```python
from build123d import *

# Parameters (mm, degrees)
F0_W     = 60
F0_H     = 60
F1_DEPTH = 7
F2_R     = 5
F3_R     = 2.1
F4_DEPTH = 25
F5_DEPTH = 3.3
F6_R     = 1
F7_DEPTH = 25
F8_R     = 1


# Not quite as in the source:
# - a feature names something its author has since deleted; it is built from what else it names


with BuildPart() as f1:
    # F0 (on Top) → F1 (new body)
    with BuildSketch(Plane.XY):
        Rectangle(F0_W, F0_H)
    extrude(amount=-F1_DEPTH)

    # F2
    f2_edges = [f1.edges().sort_by_distance(p)[0] for p in [
        (-30, 30, -3.5),
        (30, 30, -3.5),
        (30, -30, -3.5),
        (-30, -30, -3.5),
    ]]
    fillet(f2_edges, radius=F2_R)

    # F3 (on face) → F4 (cut)
    with BuildSketch(Plane.XY):
        with BuildLine():
            Line((-17, 17.9), (-17, 22.1))
            ThreePointArc((-17, 22.1), (-19.1, 20), (-17, 17.9))
        make_face()
        with BuildLine():
            ThreePointArc((-17, 17.9), (-15.5150757595, 18.5150757595), (-14.9, 20))
            ThreePointArc((-14.9, 20), (-15.5150757595, 21.4849242405), (-17, 22.1))
            Line((-17, 22.1), (-17, 17.9))
        make_face()
        with Locations((17, 20)):
            Circle(F3_R)
        with Locations((17, -20)):
            Circle(F3_R)
        with BuildLine():
            Line((-17, -22.1), (-17, -17.9))
            ThreePointArc((-17, -17.9), (-19.1, -20), (-17, -22.1))
        make_face()
        with BuildLine():
            ThreePointArc((-17, -22.1), (-15.5150757595, -21.4849242405), (-14.9, -20))
            ThreePointArc((-14.9, -20), (-15.5150757595, -18.5150757595), (-17, -17.9))
            Line((-17, -17.9), (-17, -22.1))
        make_face()
    extrude(amount=-F4_DEPTH, mode=Mode.SUBTRACT)

    # F3 (on face) → F5 (cut)
    with BuildSketch(Plane.XY):
        with BuildLine():
            ThreePointArc((-17, 17.9), (-19.1, 20), (-17, 22.1))
            Line((-17, 22.1), (-17, 23.6))
            Line((-17, 23.6), (-19.0784609691, 23.6))
            Line((-19.0784609691, 23.6), (-21.1569219382, 20))
            Line((-21.1569219382, 20), (-19.0784609691, 16.4))
            Line((-19.0784609691, 16.4), (-17, 16.4))
            Line((-17, 16.4), (-17, 17.9))
        make_face()
        with BuildLine():
            ThreePointArc((-17, 22.1), (-15.5150757595, 21.4849242405), (-14.9, 20))
            ThreePointArc((-14.9, 20), (-15.5150757595, 18.5150757595), (-17, 17.9))
            Line((-17, 17.9), (-17, 16.4))
            Line((-17, 16.4), (-14.9215390309, 16.4))
            Line((-14.9215390309, 16.4), (-12.8430780618, 20))
            Line((-12.8430780618, 20), (-14.9215390309, 23.6))
            Line((-14.9215390309, 23.6), (-17, 23.6))
            Line((-17, 23.6), (-17, 22.1))
        make_face()
        Polygon((19.0784609691, 23.6), (14.9215390309, 23.6), (12.8430780618, 20), (14.9215390309, 16.4), (19.0784609691, 16.4), (21.1569219382, 20), align=None)
        with Locations((17, 20)):
            Circle(F3_R, mode=Mode.SUBTRACT)
        with BuildLine():
            ThreePointArc((-17, -22.1), (-19.1, -20), (-17, -17.9))
            Line((-17, -17.9), (-17, -16.4))
            Line((-17, -16.4), (-19.0784609691, -16.4))
            Line((-19.0784609691, -16.4), (-21.1569219382, -20))
            Line((-21.1569219382, -20), (-19.0784609691, -23.6))
            Line((-19.0784609691, -23.6), (-17, -23.6))
            Line((-17, -23.6), (-17, -22.1))
        make_face()
        with BuildLine():
            ThreePointArc((-17, -17.9), (-15.5150757595, -18.5150757595), (-14.9, -20))
            ThreePointArc((-14.9, -20), (-15.5150757595, -21.4849242405), (-17, -22.1))
            Line((-17, -22.1), (-17, -23.6))
            Line((-17, -23.6), (-14.9215390309, -23.6))
            Line((-14.9215390309, -23.6), (-12.8430780618, -20))
            Line((-12.8430780618, -20), (-14.9215390309, -16.4))
            Line((-14.9215390309, -16.4), (-17, -16.4))
            Line((-17, -16.4), (-17, -17.9))
        make_face()
        Polygon((19.0784609691, -23.6), (21.1569219382, -20), (19.0784609691, -16.4), (14.9215390309, -16.4), (12.8430780618, -20), (14.9215390309, -23.6), align=None)
        with Locations((17, -20)):
            Circle(F3_R, mode=Mode.SUBTRACT)
    extrude(amount=-F5_DEPTH, mode=Mode.SUBTRACT)

    # F6
    f6_edges = [f1.edges().sort_by_distance(p)[0] for p in [
        (30, 0, 0),
        (0, 30, 0),
        (-30, 0, 0),
        (0, -30, 0),
        (-28.535534, -28.535534, 0),
        (28.535534, -28.535534, 0),
        (28.535534, 28.535534, 0),
        (-28.535534, 28.535534, 0),
    ]]
    fillet(f6_edges, radius=F6_R)

    # F3 (on face) → F7 (cut)
    with BuildSketch(Plane.XY):
        Polygon((-5.3375245624, 20), (-6.2035499662, 18.5), (-10.3027368774, 11.4), (-11.1687622812, 9.9), (-12.9008130888, 9.9), (-21.0991869112, 9.9), (-21.0991869112, -9.9), (-12.9008130888, -9.9), (-11.1687622812, -9.9), (-10.3027368774, -11.4), (-6.2035499662, -18.5), (-5.3375245624, -20), (5.3375245624, -20), (6.2035499662, -18.5), (10.3027368774, -11.4), (11.1687622812, -9.9), (12.9008130888, -9.9), (21.0991869112, -9.9), (21.0991869112, 9.9), (12.9008130888, 9.9), (11.1687622812, 9.9), (10.3027368774, 11.4), (6.2035499662, 18.5), (5.3375245624, 20), (0, 20), align=None)
    extrude(amount=-F7_DEPTH, mode=Mode.SUBTRACT)

    # F8
    f8_edges = [f1.edges().sort_by_distance(p)[0] for p in [
        (-16.133975, 9.9, 0),
        (-21.099187, 0, 0),
        (-8.253143, 14.95, 0),
        (0, 20, 0),
        (8.253143, 14.95, 0),
        (16.133975, 9.9, 0),
        (21.099187, 0, 0),
        (16.133975, -9.9, 0),
        (8.253143, -14.95, 0),
        (0, -20, 0),
        (-8.253143, -14.95, 0),
        (-16.133975, -9.9, 0),
        (-11.168762, 9.9, -3.5),
        (-5.337525, 20, -3.5),
        (5.337525, 20, -3.5),
        (11.168762, 9.9, -3.5),
        (21.099187, 9.9, -3.5),
        (21.099187, -9.9, -3.5),
        (11.168762, -9.9, -3.5),
        (5.337525, -20, -3.5),
        (-5.337525, -20, -3.5),
        (-11.168762, -9.9, -3.5),
        (-21.099187, -9.9, -3.5),
        (-21.099187, 9.9, -3.5),
    ]]
    fillet(f8_edges, radius=F8_R)


solid = f1.part
```
Read the model definition and answer for the solid it produces. Units are mm, in the model's axes. A direction names the side the tool comes from. Coordinates: 2 decimals unless noted, no trailing zeros. Order: outer loops, then holes, each group sorted by start corner. A loop starts at its lowest first (then second) coordinate and runs counter-clockwise, first axis right, second up. Notation, with made-up numbers: (52, 75.5) - (83, 75.5) arc R23 cw to (83, 84.5) - close; hole circle Ø1 at (27.5, -29). An arc over 180 degrees is marked (long way). Answer as a JSON object with one key per item and string values. Group by question number.
Item 1: Section A-A (y = 7) is taken. Give the vertices of the cut face in (x, z).
Item 2: Section C-C (z = -2.25) is taken. State how many separate pieces and enclosed holes the cut face has, plus the area to 3 significant figures.
Item 3: The mould has two halves that part along X. Classify faces 1 (the face through (0, 30, -4)), 2 (the face through (-17, 23.6, -2)), 3 (the face through (29, 28, -4)): +X half, -X half, draft (parallel to the pull), parting line (faces both ways), or undercut.
Item 4: Consider probe 1 along Y at (x, z) = (17, -4.85); probe 2 along X at (y, z) = (6, -6.5); probe 3 along Y at (x, z) = (2, -4.25). Determine where each line is inside the solid, lowest interval first. Write a range as from..to.
Item 5: A tool of negligible diameter and unlimited length cuts with its end or side. For faces 4 (the face through (-15, 18, -3.3)), 5 (the face through (-16, -9.9, -4)), 6 (the face through (28, -29, -4)), from which of +Z, -Z, +X, -X, +Y, -Y can it reach the whole face along a straight path? Write none if from no direction.
Item 6: Section B-B (x = 17) is taken. Give the vertices of the cut face in (y, z).
Item 7: A flat-ended cylindrical pin translates along its axis: P1, Ø3.5, axis at x = 16, y = 21.5, coming from the +Z side. Find the tip coordinate at first contact, or state that the pin passes through.
Results are:
{
 "1": {"outline": "(-30, -7) - (-21.1, -7) - (-21.1, -1) arc R1 ccw to (-22.1, 0) - (-29, 0) arc R1 ccw to (-30, -1) - close; (21.1, -7) - (30, -7) - (30, -1) arc R1 ccw to (29, 0) - (22.1, 0) arc R1 ccw to (21.1, -1) - close"},
 "2": {"separate pieces": "1", "enclosed holes": "5", "area": "2,230 mm^2"},
 "3": {"face 1": "draft", "face 2": "undercut", "face 3": "+X half"},
 "4": {"probe 1": "y = -30..-22.1, -17.9..-9.9, 9.9..17.9, 22.1..30", "probe 2": "x = -30..-21.1, 21.1..30", "probe 3": "y = -30..-20, 20..30"},
 "5": {"face 4": "+Z", "face 5": "+Z, -Z", "face 6": "+Z, -Z, +X, -Y"},
 "6": {"outline": "(-30, -7) - (-22.1, -7) - (-22.1, -3.3) - (-23.6, -3.3) - (-23.6, 0) - (-29, 0) arc R1 ccw to (-30, -1) - close; (-17.9, -7) - (-9.9, -7) - (-9.9, -1) arc R1 ccw to (-10.9, 0) - (-16.4, 0) - (-16.4, -3.3) - (-17.9, -3.3) - close; (9.9, -7) - (17.9, -7) - (17.9, -3.3) - (16.4, -3.3) - (16.4, 0) - (10.9, 0) arc R1 ccw to (9.9, -1) - close; (22.1, -7) - (30, -7) - (30, -1) arc R1 ccw to (29, 0) - (23.6, 0) - (23.6, -3.3) - (22.1, -3.3) - close"},
 "7": {"P1": "stops at z = -3.3"}
}
